```python
from build123d import *

# Parameters (mm, degrees)
SALIENTE_EXTRUIR1_DEPTH = 5
CROQUIS3_R              = 9
SALIENTE_EXTRUIR2_DEPTH = 5


with BuildPart() as part:
    # Croquis1 → Saliente-Extruir1 (new body)
    with BuildSketch(Plane.XY):
        with BuildLine():
            Line((42, 4.6), (-42, 4.6))
            Line((-42, 4.6), (-42, 1.488620272))
            ThreePointArc((-42, 1.488620272), (-41.136537684, -1.59186368), (-40.04747183, -4.6))
            Line((-40.04747183, -4.6), (-5.5, -4.6))
            Line((-5.5, -4.6), (-5.5, -9.6))
            ThreePointArc((-5.5, -9.6), (0.5, -15.6), (6.5, -9.6))
            Line((6.5, -9.6), (6.5, -4.6))
            Line((6.5, -4.6), (40.04747183, -4.6))
            ThreePointArc((40.04747183, -4.6), (41.136537684, -1.59186368), (42, 1.488620272))
            Line((42, 1.488620272), (42, 4.6))
        make_face()
        with BuildLine():
            Line((-3.5, -1.6), (-37, -1.6))
            Line((-37, -1.6), (-37, 1.6))
            Line((-37, 1.6), (37, 1.6))
            Line((37, 1.6), (37, -1.6))
            Line((37, -1.6), (4.5, -1.6))
            Line((4.5, -1.6), (4.5, -4.6))
            Line((4.5, -4.6), (4.5, -5.127864045))
            Line((4.5, -5.127864045), (4.5, -8.163859338))
            Line((4.5, -8.163859338), (4.5, -9.6))
            ThreePointArc((4.5, -9.6), (0.5, -13.6), (-3.5, -9.6))
            Line((-3.5, -9.6), (-3.5, -8.163859338))
            Line((-3.5, -8.163859338), (-3.5, -5.127864045))
            Line((-3.5, -5.127864045), (-3.5, -4.6))
            Line((-3.5, -4.6), (-3.5, -1.6))
        make_face(mode=Mode.SUBTRACT)
    extrude(amount=SALIENTE_EXTRUIR1_DEPTH)

    # Croquis3 → Saliente-Extruir2 (add)
    with BuildSketch(Plane.XY):
        with BuildLine():
            Line((6.5, -4.6), (40.04747183, -4.6))
            ThreePointArc((40.04747183, -4.6), (26.783164421, -22.295458451), (6.5, -31.108195935))
            Line((6.5, -31.108195935), (6.5, -35.6))
            Line((6.5, -35.6), (-5.5, -35.6))
            Line((-5.5, -35.6), (-5.5, -31.248453881))
            ThreePointArc((-5.5, -31.248453881), (-9.599739244, -30.51988849), (-13.610290225, -29.4))
            ThreePointArc((-13.610290225, -29.4), (-29.555859947, -19.907001489), (-40.04747183, -4.6))
            Line((-40.04747183, -4.6), (-5.5, -4.6))
            Line((-5.5, -4.6), (-5.5, -9.6))
            ThreePointArc((-5.5, -9.6), (0.5, -15.6), (6.5, -9.6))
            Line((6.5, -9.6), (6.5, -4.6))
        make_face()
        with Locations((-18.164580145, -15.2118728)):
            Circle(CROQUIS3_R, mode=Mode.SUBTRACT)
        with Locations((18.164580145, -15.2118728)):
            Circle(CROQUIS3_R, mode=Mode.SUBTRACT)
    extrude(amount=SALIENTE_EXTRUIR2_DEPTH)


solid = part.part
```
Geometry check sheet. Reference: the model listing, model coordinates, mm. A direction names the side the tool comes from. Round coordinates to 2 decimals unless told otherwise and drop trailing zeros. Order: outer loops, then holes, each group sorted by start corner. A loop starts at its lowest first (then second) coordinate and runs counter-clockwise, first axis right, second up. Notation, with made-up numbers: M 63.25,-25.5 L 115.25,-25.5 A10 cw 115.25,-14.5 Z; hole C -27.5,15.5 d4. An arc over 180 degrees is marked long. Answer as CSV lines item,"result".
1) Tool access check on faces 1 (the face through (1, 4.6, 2)), 2 (the face through (-37, 0, 2)), 3 (the face through (6.5, -33, 2)). Record the directions out of +Z, -Z, +X, -X, +Y, -Y that give a thin tool (end or side, any length) a straight path to the whole face; none if there is none.
Entries:
face 1,"+Z, -Z, +X, -X, +Y"
face 2,"+Z, -Z"
face 3,"+Z, -Z, +X, -Y"
2) Sectioned sample at C-C on x = -18. Record the cut outline in (y, z), and give its area (3 significant figures).
Entries:
outline,"M -27.67,0 L -24.21,0 L -24.21,5 L -27.67,5 Z; M -6.21,0 L -1.6,0 L -1.6,5 L -6.21,5 Z; M 1.6,0 L 4.6,0 L 4.6,5 L 1.6,5 Z"
area,"55.4 mm2"
3) Thickness scan on probe 1 along Y at (x, z) = (12, 2.9); probe 2 along X at (y, z) = (-20, 3.4); probe 3 along Y at (x, z) = (-18, 2.8). Record the ranges inside material, lowest first. Write a range as [from, to].
Entries:
probe 1,"[-29.9, -21.77], [-8.65, -1.6], [1.6, 4.6]"
probe 2,"[-29.46, -25.79], [-10.54, 10.54], [25.79, 29.46]"
probe 3,"[-27.67, -24.21], [-6.21, -1.6], [1.6, 4.6]"
4) Mould release check, pull along X, two halves, no side actions. Record for faces 4 (the face through (42, 3, 2)), 5 (the face through (-20, -1.6, 2)), 6 (the face through (1, -15, 5)), 7 (the face through (-5.5, -33, 2)): +X half, -X half, draft (parallel to the pull), parting line (faces both ways), or undercut.
Entries:
face 4,"+X half"
face 5,"undercut"
face 6,"draft"
face 7,"-X half"
5) Gauge pin test, flat ends, axial feed: pin 1 Ø23.5 at (x, y) = (18.16, -15.21) entering from +Z; pin 2 Ø1 at (y, z) = (0.5, 3) entering from +X; pin 3 Ø2.5 at (x, z) = (-7.5, 3) entering from -Y; pin 4 Ø1.3 at (y, z) = (-34.5, 1.5) entering from -X. Record the tip position at first contact, or that the pin passes through.
Entries:
pin 1,"z = 5"
pin 2,"x = 41.88"
pin 3,"y = -31.15"
pin 4,"x = -5.5"
6) Sectioned sample at B-B on z = 3.85. Record the cut outline in (x, y), and give its area (3 significant figures).
Entries:
outline,"M -42,1.49 A43.2 ccw -5.5,-31.25 L -5.5,-35.6 L 6.5,-35.6 L 6.5,-31.11 A43.2 ccw 42,1.49 L 42,4.6 L -42,4.6 Z; hole M -37,-1.6 L -3.5,-1.6 L -3.5,-9.6 A4 ccw 4.5,-9.6 L 4.5,-1.6 L 37,-1.6 L 37,1.6 L -37,1.6 Z; hole C -18.16,-15.21 d18; hole C 18.16,-15.21 d18"
area,"1,540 mm2"
7) Sectioned sample at D-D on y = -17.5. Record the cut outline in (x, z), and give its area (3 significant figures).
Entries:
outline,"M -31.93,0 L -26.87,0 L -26.87,5 L -31.93,5 Z; M -9.46,0 L 9.46,0 L 9.46,5 L -9.46,5 Z; M 26.87,0 L 31.93,0 L 31.93,5 L 26.87,5 Z"
area,"145 mm2"
8) Sectioned sample at A-A on x = 0.5. Record the cut outline in (y, z), and give its area (3 significant figures).
Entries:
outline,"M -35.6,0 L -13.6,0 L -13.6,5 L -35.6,5 Z; M 1.6,0 L 4.6,0 L 4.6,5 L 1.6,5 Z"
area,"125 mm2"
